The model under review builds one solid part; all positions refer to its coordinate system, in mm. Face numbers are marked on the shaded views. A direction names the side the tool comes from. Round coordinates to 2 decimals unless told otherwise and drop trailing zeros. Loops run counter-clockwise (first coordinate to the right, second up) from the corner with the lowest first, then second, coordinate; pieces in that order, holes last. Notation, with made-up numbers: M 44.25,46.25 L 90.25,46.25 A19 ccw 90.25,57.25 Z; hole C -11.75,-21.75 d7. An arc over 180 degrees is marked long. Answer as a JSON object with one key per item and string values. Group by question number.
Item 1: Tool access review of the marked faces 4 and 5: name each direction out of +Z, -Z, +X, -X, +Y, -Y from which nothing blocks a thin tool from reaching the whole face with its end or side.
Item 2: Consider section D-D (z = 3.25). Give the boundary of the cut face in (x, y), and give its area (3 significant figures).
Item 3: The part is to be moulded in two halves that separate along Z. For the marked faces 1, 2 and 3, say which applies: +Z half, -Z half, draft (parallel to the pull), parting line (faces both ways), or undercut.
Item 4: To check wall thickness, follow line 1 (Z direction, x = 71.5, y = -4.25); line 2 (Y direction, x = 5.5, z = 1.75); line 3 (Y direction, x = 49, z = -4.25). State the ranges of each line that lie inside material, in increasing order.
Item 5: Consider section C-C (z = 0). Give the boundary of the cut face in (x, y), and give its area (3 significant figures).
Item 6: Consider section A-A (x = 65). Give the boundary of the cut face in (y, z), and give its area (3 significant figures).
Item 7: Consider section B-B (y = -10). Give the boundary of the cut face in (x, z), and give its area (3 significant figures).
Autodesk Inventor part; units mm, degrees
ref_plane "YZ Plane" through (0, 0, 0) normal (1, 0, 0) x (0, 1, 0)
ref_plane "XZ Plane" through (0, 0, 0) normal (0, 1, 0) x (-1, 0, 0)
ref_plane "XY Plane" through (0, 0, 0) normal (0, 0, 1) x (1, 0, 0)
sketch "スケッチ1" plane through (0, 0, 0) normal (1, 0, 0) x (0, 1, 0)
  line L0 (5, 5) -> (-25, 5)
  line L1 (-25, 5) -> (-25, -5)
  line L2 (-25, -5) -> (5, -5)
  line L3 (5, -5) -> (5, 5)
  line L4 (4, 4) -> (-24, 4)
  line L5 (-24, 4) -> (-24, -4)
  line L6 (-24, -4) -> (4, -4)
  line L7 (4, -4) -> (4, 4)
  point P0 (0, 0)
  dimension "d0" = 1
  dimension "d1" = 1
  dimension "d2" = 1
  dimension "d3" = 1
  dimension "d4" = 10
  dimension "d5" = 30
  dimension "d6" = 5
  dimension "d7" = 5
extrude "押し出し1" add sketch "スケッチ1" along normal blind 80
sketch "スケッチ2" plane through (0, -25, -5) normal (0, 0, -1) x (-1, 0, 0)
  circle A0 centre (-40, 15) radius 10
  line L0 (0, 30) -> (-80, 30)
  line L1 (0, 0) -> (-80, 0)
  line L2 (0, 0) -> (0, 30)
  line L3 (-80, 0) -> (-80, 30)
  circle A1 centre (-49, 24) radius 1.5
  circle A2 centre (-31, 24) radius 1.5
  circle A3 centre (-49, 6) radius 1.5
  circle A4 centre (-31, 6) radius 1.5
  point P0 (0, 25)
  dimension "d10" = 20
  dimension "d11" = 15
  dimension "d12" = 15
  dimension "d13" = 40
  dimension "d14" = 40
  dimension "d15" = 3
  dimension "d16" = 3
  dimension "d17" = 3
  dimension "d18" = 3
  dimension "d19" = 18
  dimension "d20" = 0
  dimension "d21" = 18
  dimension "d22" = 18
  dimension "d23" = 18
  dimension "d24" = 0
  dimension "d25" = 9
  dimension "d26" = 9
  dimension "d27" = 9
  dimension "d28" = 9
  dimension "d29" = 9
  dimension "d30" = 9
  dimension "d31" = 9
extrude "押し出し2" cut sketch "スケッチ2" against normal blind 60 contours A0 | A1 | A2 | A3 | A4
sketch "スケッチ3" plane through (0, -25, -5) normal (0, -1, 0) x (1, 0, 0)
  circle A0 centre (5, 5) radius 1.5
  circle A1 centre (75, 5) radius 1.5
  line L0 (0, 10) -> (0, 0)
  line L1 (0, 0) -> (80, 0)
  line L2 (80, 10) -> (80, 0)
  point P0 (0, 5)
  dimension "d34" = 5
  dimension "d35" = 5
  dimension "d36" = 3
  dimension "d37" = 5
  dimension "d38" = 3
  dimension "d39" = 5
extrude "押し出し3" cut sketch "スケッチ3" against normal blind 60
sketch "スケッチ4" plane through (0, -25, -5) normal (0, 0, -1) x (-1, 0, 0)
  circle A0 centre (-15, 5) radius 1.5
  circle A1 centre (-15, 25) radius 1.5
  circle A2 centre (-65, 5) radius 1.5
  circle A3 centre (-65, 25) radius 1.5
  line L0 (0, 0) -> (0, 30)
  line L1 (-80, 0) -> (-80, 30)
  line L2 (0, 0) -> (-80, 0)
  line L3 (0, 30) -> (-80, 30)
  point P0 (0, 25)
  dimension "d42" = 3
  dimension "d43" = 3
  dimension "d44" = 15
  dimension "d45" = 15
  dimension "d46" = 15
  dimension "d47" = 15
  dimension "d48" = 3
  dimension "d49" = 3
  dimension "d50" = 5
  dimension "d51" = 5
  dimension "d52" = 5
  dimension "d53" = 5
extrude "押し出し4" cut sketch "スケッチ4" against normal blind 43 contours A0 | A1 | A2 | A3
properties part number "モーターパーツ１" material "アルミニウム 6061"
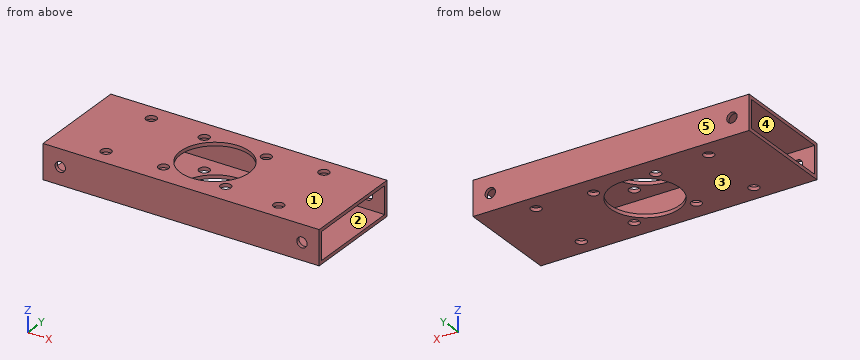
Geometry results:
{
 "1": {"face 4": "+X, -X", "face 5": "+Z, -Z, +X, -X, +Y"},
 "2": {"outline": "M 0,-25 L 80,-25 L 80,-24 L 0,-24 Z; M 0,4 L 80,4 L 80,5 L 0,5 Z", "area": "160 mm^2"},
 "3": {"face 1": "+Z half", "face 2": "undercut", "face 3": "-Z half"},
 "4": {"line 1": "z = -5 to -4, 4 to 5", "line 2": "y = -25 to -24, 4 to 5", "line 3": "y = -25 to -20.5, -17.5 to -14.36, -5.64 to -2.5, 0.5 to 5"},
 "5": {"outline": "M 0,-25 L 3.5,-25 L 3.5,-24 L 0,-24 Z; M 0,4 L 3.5,4 L 3.5,5 L 0,5 Z; M 6.5,-25 L 73.5,-25 L 73.5,-24 L 6.5,-24 Z; M 6.5,4 L 73.5,4 L 73.5,5 L 6.5,5 Z; M 76.5,-25 L 80,-25 L 80,-24 L 76.5,-24 Z; M 76.5,4 L 80,4 L 80,5 L 76.5,5 Z", "area": "148 mm^2"},
 "6": {"outline": "M -25,-5 L -21.5,-5 L -21.5,-4 L -24,-4 L -24,4 L -21.5,4 L -21.5,5 L -25,5 Z; M -18.5,-5 L -1.5,-5 L -1.5,-4 L -18.5,-4 Z; M -18.5,4 L -1.5,4 L -1.5,5 L -18.5,5 Z; M 1.5,-5 L 5,-5 L 5,5 L 1.5,5 L 1.5,4 L 4,4 L 4,-4 L 1.5,-4 Z", "area": "64.0 mm^2"},
 "7": {"outline": "M 0,-5 L 30,-5 L 30,-4 L 0,-4 Z; M 0,4 L 30,4 L 30,5 L 0,5 Z; M 50,-5 L 80,-5 L 80,-4 L 50,-4 Z; M 50,4 L 80,4 L 80,5 L 50,5 Z", "area": "120 mm^2"}
}
